Verification items for the finished model (mm, model axes). Round coordinates to 2 decimals unless told otherwise and drop trailing zeros. Loops run counter-clockwise (first coordinate to the right, second up) from the corner with the lowest first, then second, coordinate; pieces in that order, holes last. Notation, with made-up numbers: M 47.5,52 L 71.5,52 A23 cw 71.5,85 Z; hole C 28,88 d8. An arc over 180 degrees is marked long. One line per item, written item: value.
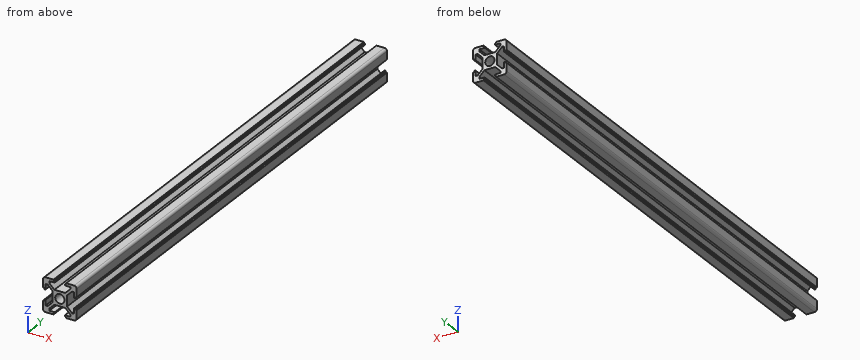
from build123d import *

# Parameters (mm, degrees)
SKETCH1_R           = 2.75
BOSS_EXTRUDE1_DEPTH = 300


with BuildPart() as part:
    # Sketch1 → Boss-Extrude1 (new body)
    with BuildSketch(Plane.XZ):
        with BuildLine():
            Line((-8.5, -10), (-3.75, -10))
            Line((-3.75, -10), (-3.75, -9.65))
            ThreePointArc((-3.75, -9.65), (-3.632842712, -9.367157288), (-3.35, -9.25))
            Line((-3.35, -9.25), (-3, -9.25))
            Line((-3, -9.25), (-3, -8.5))
            Line((-3, -8.5), (-6.2, -8.5))
            Line((-6.2, -8.5), (-6.2, -7.260660172))
            Line((-6.2, -7.260660172), (-3.239339828, -4.3))
            Line((-3.239339828, -4.3), (3.239339828, -4.3))
            Line((3.239339828, -4.3), (6.2, -7.260660172))
            Line((6.2, -7.260660172), (6.2, -8.5))
            Line((6.2, -8.5), (3, -8.5))
            Line((3, -8.5), (3, -9.25))
            Line((3, -9.25), (3.35, -9.25))
            ThreePointArc((3.35, -9.25), (3.632842712, -9.367157288), (3.75, -9.65))
            Line((3.75, -9.65), (3.75, -10))
            Line((3.75, -10), (8.5, -10))
            ThreePointArc((8.5, -10), (9.560660172, -9.560660172), (10, -8.5))
            Line((10, -8.5), (10, -3.75))
            Line((10, -3.75), (9.65, -3.75))
            ThreePointArc((9.65, -3.75), (9.367157288, -3.632842712), (9.25, -3.35))
            Line((9.25, -3.35), (9.25, -3))
            Line((9.25, -3), (8.5, -3))
            Line((8.5, -3), (8.5, -6.2))
            Line((8.5, -6.2), (7.260660172, -6.2))
            Line((7.260660172, -6.2), (4.3, -3.239339828))
            Line((4.3, -3.239339828), (4.3, 3.239339828))
            Line((4.3, 3.239339828), (7.260660172, 6.2))
            Line((7.260660172, 6.2), (8.5, 6.2))
            Line((8.5, 6.2), (8.5, 3))
            Line((8.5, 3), (9.25, 3))
            Line((9.25, 3), (9.25, 3.35))
            ThreePointArc((9.25, 3.35), (9.367157288, 3.632842712), (9.65, 3.75))
            Line((9.65, 3.75), (10, 3.75))
            Line((10, 3.75), (10, 8.5))
            ThreePointArc((10, 8.5), (9.560660172, 9.560660172), (8.5, 10))
            Line((8.5, 10), (3.75, 10))
            Line((3.75, 10), (3.75, 9.65))
            ThreePointArc((3.75, 9.65), (3.632842712, 9.367157288), (3.35, 9.25))
            Line((3.35, 9.25), (3, 9.25))
            Line((3, 9.25), (3, 8.5))
            Line((3, 8.5), (6.2, 8.5))
            Line((6.2, 8.5), (6.2, 7.260660172))
            Line((6.2, 7.260660172), (3.239339828, 4.3))
            Line((3.239339828, 4.3), (-3.239339828, 4.3))
            Line((-3.239339828, 4.3), (-6.2, 7.260660172))
            Line((-6.2, 7.260660172), (-6.2, 8.5))
            Line((-6.2, 8.5), (-3, 8.5))
            Line((-3, 8.5), (-3, 9.25))
            Line((-3, 9.25), (-3.35, 9.25))
            ThreePointArc((-3.35, 9.25), (-3.632842712, 9.367157288), (-3.75, 9.65))
            Line((-3.75, 9.65), (-3.75, 10))
            Line((-3.75, 10), (-8.5, 10))
            ThreePointArc((-8.5, 10), (-9.560660172, 9.560660172), (-10, 8.5))
            Line((-10, 8.5), (-10, 3.75))
            Line((-10, 3.75), (-9.65, 3.75))
            ThreePointArc((-9.65, 3.75), (-9.367157288, 3.632842712), (-9.25, 3.35))
            Line((-9.25, 3.35), (-9.25, 3))
            Line((-9.25, 3), (-8.5, 3))
            Line((-8.5, 3), (-8.5, 6.2))
            Line((-8.5, 6.2), (-7.260660172, 6.2))
            Line((-7.260660172, 6.2), (-4.3, 3.239339828))
            Line((-4.3, 3.239339828), (-4.3, -3.239339828))
            Line((-4.3, -3.239339828), (-7.260660172, -6.2))
            Line((-7.260660172, -6.2), (-8.5, -6.2))
            Line((-8.5, -6.2), (-8.5, -3))
            Line((-8.5, -3), (-9.25, -3))
            Line((-9.25, -3), (-9.25, -3.35))
            ThreePointArc((-9.25, -3.35), (-9.367157288, -3.632842712), (-9.65, -3.75))
            Line((-9.65, -3.75), (-10, -3.75))
            Line((-10, -3.75), (-10, -8.5))
            ThreePointArc((-10, -8.5), (-9.560660172, -9.560660172), (-8.5, -10))
        make_face()
        Circle(SKETCH1_R, mode=Mode.SUBTRACT)
    extrude(amount=-BOSS_EXTRUDE1_DEPTH)


solid = part.part
(1) Depth check by flat-ended pin: pin 1 Ø1.9 at (y, z) = (187.5, -1.5) entering from -X; pin 2 Ø0.6 at (y, z) = (149.5, 9) entering from +X; pin 3 Ø6 at (x, y) = (-0.5, 251) entering from -Z. Enter the tip coordinate at first touch or a pass-through.
Completed:
pin 1: stops at x = -4.3
pin 2: stops at x = 9.99
pin 3: stops at z = -9.28
(2) Thickness scan on L1, parallel to X at y = 106.5, z = -3.25; L2, parallel to X at y = 115.5, z = -8; L3, parallel to Z at x = 0, y = 149. Record the ranges inside material, lowest first. Write a range as from..to.
Completed:
L1: x = -9.25..-8.5, -4.31..4.31, 8.5..9.25
L2: x = -10..-6.2, 6.2..10
L3: z = -4.3..-2.75, 2.75..4.3
(3) Sectioned sample at A-A on x = 0. Enter the section's corners in (y, z), and give its area (3 significant figures).
Completed:
outline: M 0,-4.3 L 300,-4.3 L 300,-2.75 L 0,-2.75 Z; M 0,2.75 L 300,2.75 L 300,4.3 L 0,4.3 Z
area: 930 mm^2
(4) Sectioned sample at B-B on z = 0. Enter the section's corners in (x, y), and give its area (3 significant figures).
Completed:
outline: M -4.3,0 L -2.75,0 L -2.75,300 L -4.3,300 Z; M 2.75,0 L 4.3,0 L 4.3,300 L 2.75,300 Z
area: 930 mm^2
